CAD build for the part. Positions are in the model's coordinates, mm. A direction names the side the tool comes from. Coordinates: 2 decimals unless noted, no trailing zeros. Write each loop counter-clockwise with the first axis right and the second up, starting at its lowest first coordinate (ties: lowest second). Pieces come first, ordered by that corner, then holes. Notation, with made-up numbers: (-15, 38) - (9, 38) arc R35 cw to (9, 72) - close; hole circle Ø3 at (-18, 53.25). An arc over 180 degrees is marked (long way). Answer in a Markdown table with one row per item. Add a question column.
Q1. Band-saw the part on C-C (z = 24). List the corners of the cut face in (x, y).
Q2. Two-plate mould, pull along X, no slides. Class faces 4 (the flat face through (14.483, 37.168, -0.028)), 5 (the flat face through (10, 2, 30)), 6 (the flat face through (26, 73, 2)): +X half, -X half, draft (parallel to the pull), parting line (faces both ways), or undercut.
Q3. Band-saw the part on B-B (x = 23). List the corners of the cut face in (y, z).
Q4. 3-axis set-ups, long thin cutter, end or side, ignore diameter. For faces 1 (the flat face through (26, 73, -2)), 2 (the flat face through (25, 126, 0)), 3 (the cylindrical face through (-4, 14, 3)): which of +Z, -Z, +X, -X, +Y, -Y reach the whole face in a straight line?
Q5. Band-saw the part on A-A (y = 86). List the corners of the cut face in (x, z).
Q6. Pin check, flat tips, straight feed: pin 1 (1 mm diameter, centred on x = -5, z = 0, fed in from +Y); pin 2 (2.5 mm diameter, centred on y = 170, z = -10.5, fed in from -X); pin 3 (4 mm diameter, centred on x = -6.5, z = 12, fed in from +Y); pin 4 (1.8 mm diameter, centred on y = 107.5, z = 10.5, fed in from +X). Stop position of each tip, or through.
Q7. Drill centre lines: line 1 along Z through (x, y) = (33, 70); line 2 along Z through (x, y) = (8, 19); line 3 along X through (y, z) = (23.5, 13). Where is each one in solid material? Low to high. Write a range as from..to.
Autodesk Inventor part; units mm, degrees
ref_plane "YZ Plane" through (0, 0, 0) normal (1, 0, 0) x (0, 1, 0)
ref_plane "XZ Plane" through (0, 0, 0) normal (0, 1, 0) x (-1, 0, 0)
ref_plane "XY Plane" through (0, 0, 0) normal (0, 0, 1) x (1, 0, 0)
sketch "Sketch1" plane through (0, 0, 0) normal (0, 1, 0) x (-1, 0, 0)
  line L0 (-15, -19.5) -> (-15, 0) construction
  line L1 (-15, 0) -> (-15, 19.5) construction
  line L2 (15, -30) -> (-35, -30)
  line L3 (-35, -30) -> (-35, 30)
  line L4 (-35, 30) -> (15, 30)
  line L5 (15, 30) -> (15, -30)
  circle A0 centre (0, 0) radius 5
  point P0 (15, 0)
  dimension "d0" = 15
  dimension "d1" = 19.5
  dimension "d2" = 60
  dimension "d3" = 50
  dimension "d4" = 20
  dimension "d22" = 10
extrude "Extrusion1" add sketch "Sketch1" along normal blind 4 contours L2 L3 L4 L5 | A0
sketch "Sketch2" plane through (0, 0, 0) normal (0, 0, 1) x (1, 0, 0)
  line L0 (35, 4) -> (-15, 4)
  line L1 (35, 4) -> (35, 200)
  line L2 (35, 200) -> (25, 200)
  line L3 (25, 200) -> (25, 49)
  line L4 (25, 49) -> (-15, 4)
  line L5 (32, 200) -> (32, 4)
  line L6 (-15, 0) -> (35, 0)
  point P0 (0, 0)
  dimension "d14" = 10
  dimension "d15" = 3
  dimension "d16" = 45
  dimension "d17" = 200
extrude "Extrusion2" add sketch "Sketch2" along normal mid plane 4 contours L0 L4 L3 L2 L5
extrude "breedte arm" add sketch "Sketch2" along normal mid plane 30 contours L0 L5 L2 L1
extrude "Extrusion4" add sketch "Sketch1" along normal blind 25 contours A0
hole "Hole2" at (0, 0, 0) at (15, 0, -19.5) at (15, 0, 19.5) direction (0, 1, 0) diameter 3.4 end through all
sketch "Sketch3" plane through (35, 0, 30) normal (1, 0, 0) x (0, 0, -1)
  line L0 (15, 200) -> (45, 200)
  line L1 (19.5, 195) -> (15, 195) construction
  line L2 (15, 200) -> (15, 4) construction
  line L3 (40.5, 195) -> (45, 195) construction
  line L4 (45, 4) -> (45, 200) construction
  point P0 (30, 0)
  point P1 (42.75, 195)
  point P2 (19.5, 182.5)
  point P3 (40.5, 182.5)
  point P4 (19.5, 170)
  point P5 (40.5, 170)
  point P6 (19.5, 157.5)
  point P7 (40.5, 157.5)
  point P8 (19.5, 145)
  point P9 (40.5, 145)
  point P10 (19.5, 132.5)
  point P11 (40.5, 132.5)
  point P12 (19.5, 120)
  point P13 (40.5, 120)
  point P14 (19.5, 107.5)
  point P15 (40.5, 107.5)
  point P16 (19.5, 95)
  point P17 (40.5, 95)
  point P18 (19.5, 82.5)
  point P19 (40.5, 82.5)
  point P20 (19.5, 70)
  point P21 (40.5, 70)
  point P22 (19.5, 57.5)
  point P23 (40.5, 57.5)
  dimension "d32" = 5
  dimension "d33" = 21
  dimension "d36" = 12.5
hole "Hole3" at (35, 195, 10.5) at (35, 195, -10.5) at (35, 182.5, -10.5) at (35, 182.5, 10.5) at (35, 170, 10.5) at (35, 170, -10.5) at (35, 157.5, -10.5) at (35, 157.5, 10.5) at (35, 145, 10.5) at (35, 145, -10.5) at (35, 132.5, -10.5) at (35, 132.5, 10.5) at (35, 120, 10.5) at (35, 120, -10.5) at (35, 107.5, -10.5) at (35, 107.5, 10.5) at (35, 95, 10.5) at (35, 95, -10.5) at (35, 82.5, 10.5) at (35, 70, 10.5) at (35, 57.5, 10.5) at (35, 57.5, -10.5) at (35, 70, -10.5) at (35, 82.5, -10.5) direction (-1, 0, 0) diameter 2.2 end through all
properties part number "camera arm"
Checked values:
| question | item | result |
|---|---|---|
| 1 | outline | (-15, 0) - (35, 0) - (35, 4) - (-15, 4) - close |
| 2 | face 4 | -X half |
| 2 | face 5 | draft |
| 2 | face 6 | undercut |
| 3 | outline | (0, -30) - (4, -30) - (4, -2) - (46.75, -2) - (46.75, 2) - (4, 2) - (4, 30) - (0, 30) - close |
| 4 | face 1 | -Z, +Y |
| 4 | face 2 | +Z, -Z, -X, +Y |
| 4 | face 3 | +Y |
| 5 | outline | (25, -2) - (32, -2) - (32, -15) - (35, -15) - (35, 15) - (32, 15) - (32, 2) - (25, 2) - close |
| 6 | pin 1 | stops at y = 25 |
| 6 | pin 2 | stops at x = 32 |
| 6 | pin 3 | stops at y = 4 |
| 6 | pin 4 | passes through |
| 7 | line 1 | z = -15..-11.6, -9.4..9.4, 11.6..15 |
| 7 | line 2 | z = -2..2 |
| 7 | line 3 | x = 32..35 |
